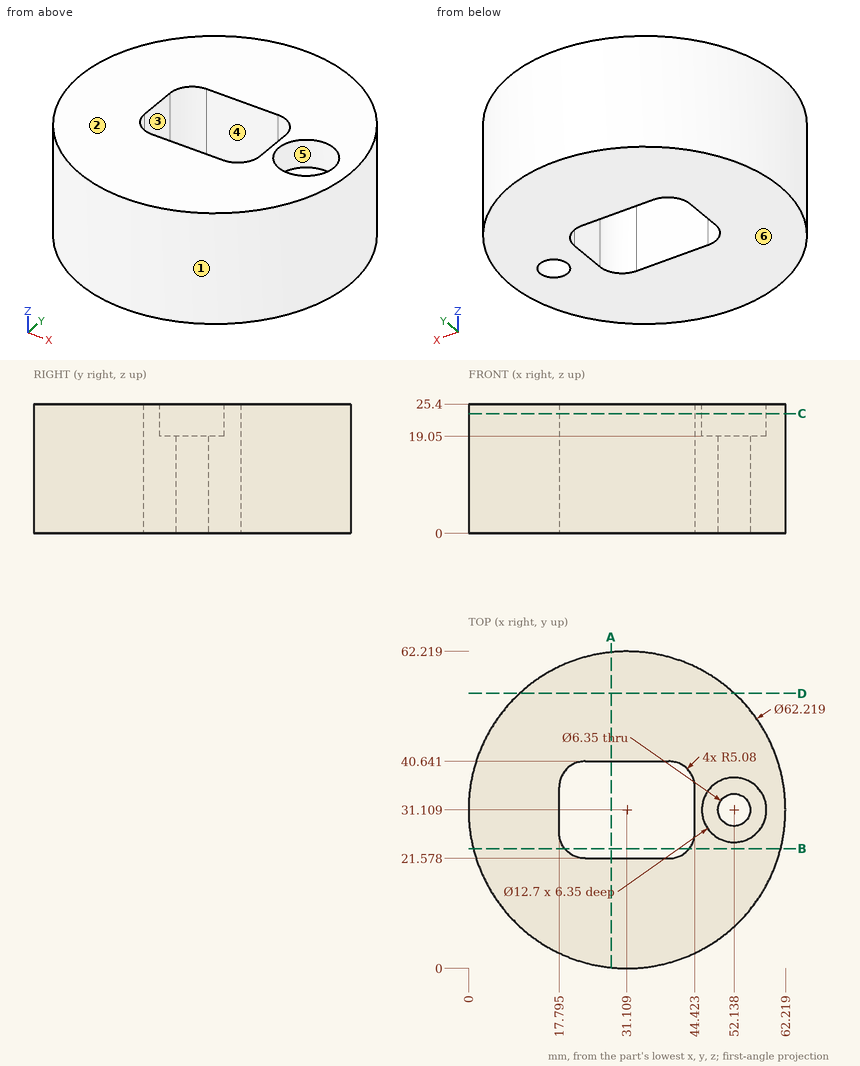
Here's the drawing with two shaded views (mm, measured from the low corner). I have some questions. A direction names the side the tool comes from. Coordinates: 2 decimals unless noted, no trailing zeros. Loops run counter-clockwise (first coordinate to the right, second up) from the corner with the lowest first, then second, coordinate; pieces in that order, holes last. Notation, with made-up numbers: (54.25, 86.25) -> (87.25, 86.25) arc R20 cw to (87.25, 99.25) -> close; hole circle Ø2 at (51, -11). An arc over 180 degrees is marked (long way). Answer in a Markdown table with one row per item.
(1) Will these pins go through, and if not, where does the flat tip stop? pin 1 Ø13 at (x, z) = (28, 17) entering from +Y; pin 2 Ø10 at (x, y) = (52.14, 31.11) entering from +Z; pin 3 Ø5 at (x, z) = (12.5, 20) entering from +Y; pin 4 Ø8 at (x, y) = (38.5, 33.5) entering from -Z.
Results found:
| item | result |
|---|---|
| pin 1 | stops at y = 62.22 |
| pin 2 | stops at z = 19.05 |
| pin 3 | stops at y = 57.72 |
| pin 4 | passes through |
(2) If I drill on probe 1 along X at (y, z) = (31, 6.5) (1 decimal); probe 2 along Y at (x, z) = (32, 24.25) (1 decimal); probe 3 along Y at (x, z) = (33, 22), over which ranges is the centre line in solid material (lowest first)?
Results found:
| item | result |
|---|---|
| probe 1 | x = 0 to 17.8, 44.4 to 49, 55.3 to 62.2 |
| probe 2 | y = 0 to 21.6, 40.6 to 62.2 |
| probe 3 | y = 0.06 to 21.58, 40.64 to 62.16 |
(3) For the marked faces 4, 5 and 6, which set-ups out of +Z, -Z, +X, -X, +Y, -Y let a thin tool reach every point of the face, with its end or its side?
Results found:
| item | result |
|---|---|
| face 4 | +Z, -Z |
| face 5 | +Z |
| face 6 | -Z, +X, -X, +Y, -Y |
(4) Imagine slicing it at D-D (y = 54). List the corners of the cut face in (x, z) for me (1 decimal), plus the area to 3 significant figures.
Results found:
| item | result |
|---|---|
| outline | (10, 0) -> (52.2, 0) -> (52.2, 25.4) -> (10, 25.4) -> close |
| area | 1,070 mm^2 |
(5) Imagine slicing it at A-A (x = 28). List the corners of the cut face in (y, z) for me (1 decimal), plus the area to 3 significant figures.
Results found:
| item | result |
|---|---|
| outline | (0.2, 0) -> (21.6, 0) -> (21.6, 25.4) -> (0.2, 25.4) -> close; (40.6, 0) -> (62.1, 0) -> (62.1, 25.4) -> (40.6, 25.4) -> close |
| area | 1,090 mm^2 |
(6) Imagine slicing it at B-B (y = 23.5). List the corners of the cut face in (x, z) for me (1 decimal), plus the area to 3 significant figures.
Results found:
| item | result |
|---|---|
| outline | (0.9, 0) -> (18.9, 0) -> (18.9, 25.4) -> (0.9, 25.4) -> close; (43.3, 0) -> (61.3, 0) -> (61.3, 25.4) -> (43.3, 25.4) -> close |
| area | 912 mm^2 |
(7) Thinking about a two-plate mould opening in Y: for the marked faces 1, 2 and 3, which applies, released by +Y, released by -Y, zero draft, split by the parting line, or undercut?
Results found:
| item | result |
|---|---|
| face 1 | split by the parting line |
| face 2 | zero draft |
| face 3 | undercut |
(8) Imagine slicing it at C-C (z = 23.5). Give the number of separate pieces and of enclosed holes in the cut face, plus the area to 3 significant figures.
Results found:
| item | result |
|---|---|
| separate pieces | 1 |
| enclosed holes | 2 |
| area | 2,430 mm^2 |
